Geometry: final body of the model. Coordinates: model frame, mm. Coordinates: 2 decimals unless noted, no trailing zeros. Loops run counter-clockwise (first coordinate to the right, second up) from the corner with the lowest first, then second, coordinate; pieces in that order, holes last. Notation, with made-up numbers: (68, 86) -> (79, 86) arc R22 ccw to (79, 94) -> close; hole circle Ø2 at (42, -27.75). An arc over 180 degrees is marked (long way). One line per item, written item: value. Start each with the question number.
Item 1: Section query B-B on z = 4. Return loops of the section in (x, y), then the cut area to 3 significant figures.
Item 2: Section query A-A on x = 0. Return loops of the section in (y, z), then the cut area to 3 significant figures.
Item 3: Section query C-C on y = 80. Return loops of the section in (x, z), then the cut area to 3 significant figures.
Item 4: Contact query for flat-ended pins moving along their axis: pin 1 Ø1.5 at (y, z) = (58, 2.5) entering from -X; pin 2 Ø15.5 at (x, y) = (0, 80) entering from +Z; pin 3 Ø1 at (x, z) = (65, 4) entering from +Y; pin 4 Ø2 at (x, z) = (77.5, 2.5) entering from -Y. Output: stop coordinate, or through.
Item 5: Ray query, probe 1 along Y at (x, z) = (80, 3.25); probe 2 along Y at (x, z) = (26.5, 6.75). Return the intervals inside material, ascending. Write a range as from..to.
Autodesk Inventor part; units mm, degrees
ref_plane "YZ Plane" through (0, 0, 0) normal (1, 0, 0) x (0, 1, 0)
ref_plane "XZ Plane" through (0, 0, 0) normal (0, 1, 0) x (-1, 0, 0)
ref_plane "XY Plane" through (0, 0, 0) normal (0, 0, 1) x (1, 0, 0)
sketch "Sketch2" plane through (0, 0, 0) normal (0, 0, 1) x (1, 0, 0)
  circle A0 centre (0, 0) radius 45.5
  circle A1 centre (0, 0) radius 97.5
  dimension "d25" = 91
  dimension "d27" = 195
extrude "Plate2" add sketch "Sketch2" along normal blind 8
sketch "Sketch3" plane through (0, 0, 8) normal (0, 0, 1) x (1, 0, 0)
  circle A0 centre (-80, 0) radius 8.5
  circle A1 centre (0, 0) radius 80 construction
  dimension "d28" = 160
  dimension "d15" = 17
extrude "Cut1" cut sketch "Sketch3" against normal blind 8
pattern_circular "Circular Pattern1" count 4 over 360 about axis through (0, 0, -10) along (0, 0, 1) of "Cut1"
equation "\"d17\" = Thickness"
equation "\"d14\" = Thickness"
equation "\"BendReliefWidth\" = Thickness"
equation "\"BendReliefDepth\" = 0.5 * Thickness"
equation "\"CornerReliefSize\" = 4 * Thickness"
equation "\"MinimumRemnant\" = 2 * Thickness"
equation "\"TransitionRadius\" = BendRadius"
equation "\"JacobiRadiusSize\" = BendRadius"
equation "\"GapSize\" = Thickness"
properties part number "SLM 1633 charging blind flange" material "Steel"
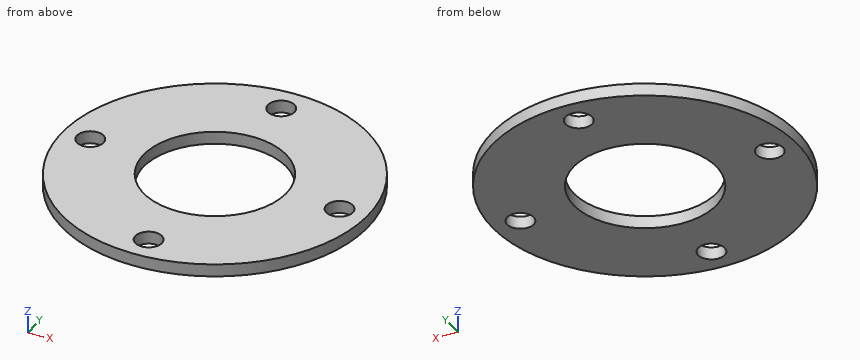
Reply:
1. outline: circle Ø195 at (0, 0); hole circle Ø17 at (-80, 0); hole circle Ø91 at (0, 0); hole circle Ø17 at (0, -80); hole circle Ø17 at (0, 80); hole circle Ø17 at (80, 0)
1. area: 22,500 mm²
2. outline: (-97.5, 0) -> (-88.5, 0) -> (-88.5, 8) -> (-97.5, 8) -> close; (-71.5, 0) -> (-45.5, 0) -> (-45.5, 8) -> (-71.5, 8) -> close; (45.5, 0) -> (71.5, 0) -> (71.5, 8) -> (45.5, 8) -> close; (88.5, 0) -> (97.5, 0) -> (97.5, 8) -> (88.5, 8) -> close
2. area: 560 mm²
3. outline: (-55.73, 0) -> (-8.5, 0) -> (-8.5, 8) -> (-55.73, 8) -> close; (8.5, 0) -> (55.73, 0) -> (55.73, 8) -> (8.5, 8) -> close
3. area: 756 mm²
4. pin 1: stops at x = -78.92
4. pin 2: passes through
4. pin 3: stops at y = 73.12
4. pin 4: stops at y = -60.45
5. probe 1: y = -55.73..-8.5, 8.5..55.73
5. probe 2: y = -93.83..-36.99, 36.99..93.83
